Work out the finished part from the listing and answer in its coordinate system (mm). Face numbers are marked on the shaded views. Coordinates: 2 decimals unless noted, no trailing zeros. Order: outer loops, then holes, each group sorted by start corner. A loop starts at its lowest first (then second) coordinate and runs counter-clockwise, first axis right, second up. Notation, with made-up numbers: (8.5, 66) -> (58.5, 66) arc R18 ccw to (58.5, 100) -> close; hole circle Ø5 at (14.5, 8). An arc over 180 degrees is marked (long way). Answer as CSV lines item,"result". Start each with the question number.
Item 1: Section A-A (y = 30) is taken. Write down the section's boundary in (x, z), then the cut area to 3 significant figures.
Item 2: Section C-C (z = 15) is taken. Write down the section's boundary in (x, y), then the cut area to 3 significant figures.
Item 3: Straight lines are drawn through the part: L1, parallel to Z at x = -23.5, y = 73.5; L2, parallel to X at y = 3, z = 5. For each, find the intervals that lie inside material, in ascending order.
Item 4: For a pull along Z with two mould halves and no side action, classify the marked faces 1, 2 and 3 as pulls with the +Z half, pulls with the -Z half, needs draft (parallel to the pull), parting line crosses it, or undercut.
Item 5: Section B-B (x = -56) is taken. Write down the section's boundary in (y, z), then the cut area to 3 significant figures.
```python
from build123d import *

# Parameters (mm, degrees)
F0_W     = 160
F0_H     = 425
F1_DEPTH = 0.5
F2_R     = 6.25
F3_DEPTH = 50
F4_W     = 160
F4_H     = 425
F5_DEPTH = 0.5


with BuildPart() as f1:
    # F0 (on Top) → F1 (new body)
    with BuildSketch(Plane.XY):
        Rectangle(F0_W, F0_H)
    extrude(amount=-F1_DEPTH)

    # F2 (on face) → F3 (join)
    with BuildSketch(Plane.XY):
        with Locations((-70, 202.5)):
            Circle(F2_R)
        with Locations((-70, 0)):
            Circle(F2_R)
        with Locations((-70, -202.5)):
            Circle(F2_R)
        with Locations((70, 202.5)):
            Circle(F2_R)
        with Locations((70, 0)):
            Circle(F2_R)
        with Locations((70, -202.5)):
            Circle(F2_R)
    extrude(amount=F3_DEPTH)

    # F4 (on face) → F5 (join)
    with BuildSketch(Plane.XY.offset(50)):
        Rectangle(F4_W, F4_H)
    extrude(amount=F5_DEPTH)


solid = f1.part
```
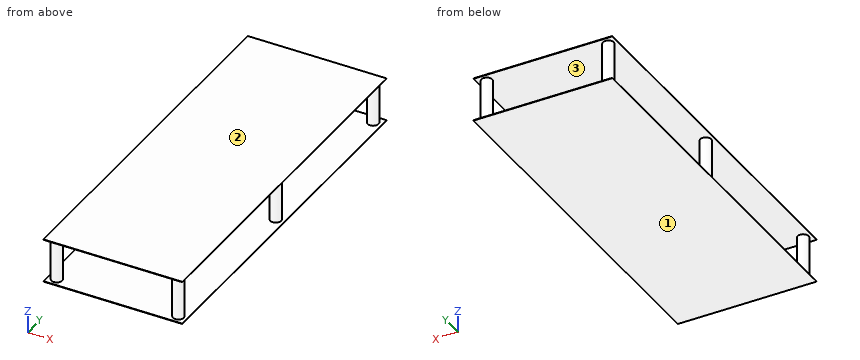
Checked values:
1,outline,"(-80, -0.5) -> (80, -0.5) -> (80, 0) -> (-80, 0) -> close; (-80, 50) -> (80, 50) -> (80, 50.5) -> (-80, 50.5) -> close"
1,area,"160 mm^2"
2,outline,"circle Ø12.5 at (-70, -202.5); circle Ø12.5 at (-70, 0); circle Ø12.5 at (-70, 202.5); circle Ø12.5 at (70, -202.5); circle Ø12.5 at (70, 0); circle Ø12.5 at (70, 202.5)"
2,area,"736 mm^2"
3,L1,"z = -0.5 to 0, 50 to 50.5"
3,L2,"x = -75.48 to -64.52, 64.52 to 75.48"
4,face 1,"pulls with the -Z half"
4,face 2,"pulls with the +Z half"
4,face 3,"undercut"
5,outline,"(-212.5, -0.5) -> (212.5, -0.5) -> (212.5, 0) -> (-212.5, 0) -> close; (-212.5, 50) -> (212.5, 50) -> (212.5, 50.5) -> (-212.5, 50.5) -> close"
5,area,"425 mm^2"
